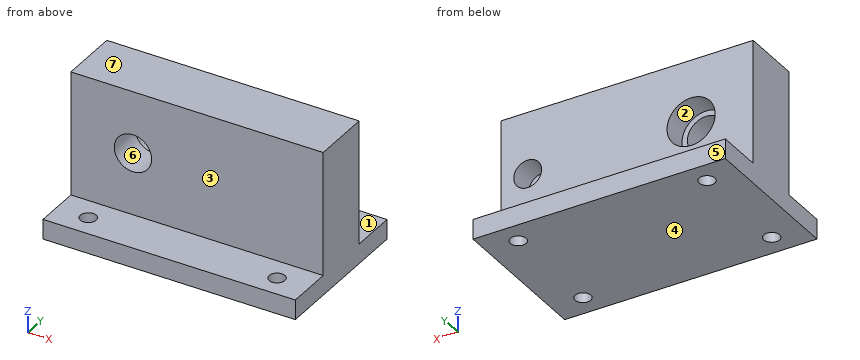
from build123d import *

# Parameters (mm, degrees)
SKETCH067_W     = 50.8
SKETCH067_H     = 30.6
PAD014_DEPTH    = 4
SKETCH068_R     = 1.6
POCKET061_DEPTH = 4.001
SKETCH069_W     = 50.8
SKETCH069_H     = 12
PAD015_DEPTH    = 25
SKETCH070_R     = 4.85
POCKET062_DEPTH = 5
SKETCH071_R     = 3.7625
POCKET063_DEPTH = 16.301
SKETCH072_R     = 2.8
POCKET064_DEPTH = 5


with BuildPart() as part:
    # Sketch067 → Pad014 (new body)
    with BuildSketch(Plane.XY):
        Rectangle(SKETCH067_W, SKETCH067_H)
    extrude(amount=PAD014_DEPTH)

    # Sketch068 (on Face6 of Pad014) → Pocket061 (cut, through all)
    with BuildSketch(Plane.XY.offset(4)):
        with Locations((19, 10.8)):
            Circle(SKETCH068_R)
        with Locations((19, -10.8)):
            Circle(SKETCH068_R)
        with Locations((-19, -10.8)):
            Circle(SKETCH068_R)
        with Locations((-19, 10.8)):
            Circle(SKETCH068_R)
    extrude(amount=-POCKET061_DEPTH, mode=Mode.SUBTRACT)

    # Sketch069 (on Face5 of Pocket061) → Pad015 (join)
    with BuildSketch(Plane.XY.offset(4)):
        Rectangle(SKETCH069_W, SKETCH069_H)
    extrude(amount=PAD015_DEPTH)

    # Sketch070 (on Face13 of Pad015) → Pocket062 (cut)
    with BuildSketch(Plane(origin=(0, 6, 0), x_dir=(-1, 0, 0), z_dir=(0, 1, 0))):
        with Locations((12.9, 16.5)):
            Circle(SKETCH070_R)
    extrude(amount=-POCKET062_DEPTH, mode=Mode.SUBTRACT)

    # Sketch071 (on Face18 of Pocket062) → Pocket063 (cut, through all)
    with BuildSketch(Plane(origin=(0, 1, 0), x_dir=(-1, 0, 0), z_dir=(0, 1, 0))):
        with Locations((12.9, 16.5)):
            Circle(SKETCH071_R)
    extrude(amount=-POCKET063_DEPTH, mode=Mode.SUBTRACT)

    # Sketch072 → Pocket064 (cut)
    with BuildSketch(Plane(origin=(0, 6, 0), x_dir=(-1, 0, 0), z_dir=(0, 1, 0))):
        with Locations((-20, 16.5)):
            Circle(SKETCH072_R)
    extrude(amount=-POCKET064_DEPTH, mode=Mode.SUBTRACT)


solid = part.part
Read the model definition and answer for the solid it produces. Units are mm, in the model's axes. Face numbers are marked on the shaded views. A direction names the side the tool comes from. Give positions to 0.01 mm unless a question says otherwise; leave off trailing zeros. Write each loop counter-clockwise with the first axis right and the second up, starting at its lowest first coordinate (ties: lowest second). Pieces come first, ordered by that corner, then holes. Notation, with made-up numbers: (64, 68.25) - (89, 68.25) arc R13 cw to (89, 77.25) - close; hole circle Ø3 at (-8, 7). An arc over 180 degrees is marked (long way). Use CSV: the item, a comma, the result in double quotes. Start each with the question number.
Item 1: The part is cut by section D-D, the plane z = 16.5. Give the vertices of the cut face in (x, y), and give its area (3 significant figures).
Item 2: Flat-ended cylindrical pins translate along their axes: P1, Ø1.9, axis at x = -19, y = 10.8, coming from the +Z side; P2, Ø5, axis at x = 19, y = 10.8, coming from the +Z side; P3, Ø8.5, axis at x = -12.9, z = 16.5, coming from the -Y side; P4, Ø6.5, axis at x = 20, z = 16.5, coming from the +Y side. Find the tip coordinate at first contact, or state that the pin passes through.
Item 3: The part is cut by section B-B, the plane z = 2.5. Give the vertices of the cut face in (x, y), and give its area (3 significant figures).
Item 4: For the marked faces 1, 2 and 3, determine the directions among +Z, -Z, +X, -X, +Y, -Y from which every point of the face is accessible in a straight line to the end or side of a thin tool.
Item 5: The part is cut by section A-A, the plane x = -19. Give the vertices of the cut face in (y, z).
Item 6: The mould has two halves that part along Z. Classify the marked faces 4, 5, 6 and 7: pulls with the +Z half, pulls with the -Z half, needs draft (parallel to the pull), parting line crosses it, or undercut.
Item 7: Consider line 1 (Y direction, x = -19, z = 1.55); line 2 (Z direction, x = -12.9, y = -0.5); line 3 (Y direction, x = -22.5, z = 23.25). Determine where each line is inside the solid, lowest interval first.
Item 8: The part is cut by section C-C, the plane x = -12.9. Give the vertices of the cut face in (y, z).
Taken from the geometry:
1,outline,"(-25.4, -6) - (-16.66, -6) - (-16.66, 1) - (-17.75, 1) - (-17.75, 6) - (-25.4, 6) - close; (-9.14, -6) - (25.4, -6) - (25.4, 6) - (22.8, 6) - (22.8, 1) - (17.2, 1) - (17.2, 6) - (-8.05, 6) - (-8.05, 1) - (-9.14, 1) - close"
1,area,"480 mm2"
2,P1,"through"
2,P2,"z = 4"
2,P3,"y = -6"
2,P4,"y = 6"
3,outline,"(-25.4, -15.3) - (25.4, -15.3) - (25.4, 15.3) - (-25.4, 15.3) - close; hole circle Ø3.2 at (-19, -10.8); hole circle Ø3.2 at (-19, 10.8); hole circle Ø3.2 at (19, -10.8); hole circle Ø3.2 at (19, 10.8)"
3,area,"1,520 mm2"
4,face 1,"+Z, +X, -X, +Y"
4,face 2,"+Y"
4,face 3,"+Z, +X, -X, -Y"
5,outline,"(-15.3, 0) - (-12.4, 0) - (-12.4, 4) - (-15.3, 4) - close; (-9.2, 0) - (9.2, 0) - (9.2, 4) - (6, 4) - (6, 29) - (-6, 29) - (-6, 4) - (-9.2, 4) - close; (12.4, 0) - (15.3, 0) - (15.3, 4) - (12.4, 4) - close"
6,face 4,"pulls with the -Z half"
6,face 5,"needs draft"
6,face 6,"undercut"
6,face 7,"pulls with the +Z half"
7,line 1,"-15.3 to -12.4, -9.2 to 9.2, 12.4 to 15.3"
7,line 2,"0 to 12.74, 20.26 to 29"
7,line 3,"-6 to 6"
8,outline,"(-15.3, 0) - (15.3, 0) - (15.3, 4) - (6, 4) - (6, 11.65) - (1, 11.65) - (1, 12.74) - (-6, 12.74) - (-6, 4) - (-15.3, 4) - close; (-6, 20.26) - (1, 20.26) - (1, 21.35) - (6, 21.35) - (6, 29) - (-6, 29) - close"
